Build history of the part. All positions in model axes, mm. Give positions to 0.01 mm unless a question says otherwise; leave off trailing zeros. Write each question's results on one line, items separated by ' | '. Start each with the question number.
1) Drill centre lines: line 1 along X through (y, z) = (1.3, 120); line 2 along Z through (x, y) = (104, 1.1). Where is each one in solid material? Low to high. Write a range as from..to.
2) Two-plate mould, pull along Y, no slides. Class faces 1 (the face through (-2, 2, -2)), 2 (the face through (-2, 0, -2)): +Y half, -Y half, draft (parallel to the pull), parting line (faces both ways), or undercut.
3) Drop a flat-ended pin along its axis: pin 1 Ø3 at (x, z) = (104, 120) entering from -Y. Give the stop position or say it passes through.
from build123d import *

# Parameters (mm, degrees)
SKETCH1_W                  = 220
SKETCH1_H                  = 280
BOSS_EXTRUDE1_DEPTH        = 2
F_3_5_3_5_DIAMETER_HOLE1_D = 3.5
FILLET1_R                  = 3


with BuildPart() as part:
    # Sketch1 → Boss-Extrude1 (new body)
    with BuildSketch(Plane(origin=(0, 0, 0), x_dir=(1, 0, 0), z_dir=(0, 1, 0))):
        Rectangle(SKETCH1_W, SKETCH1_H)
    extrude(amount=BOSS_EXTRUDE1_DEPTH)

    # Ø3.5 (3.5) Diameter Hole1 (through all)
    with Locations(Plane(origin=(0, 2, 0), x_dir=(1, 0, 0), z_dir=(0, 1, 0))):
        with Locations((-104, -120), (104, -120), (104, 120), (-104, 120), (104, 0), (-104, 0)):
            Hole(F_3_5_3_5_DIAMETER_HOLE1_D / 2)

    # Fillet1
    fillet1_edges = [part.edges().sort_by_distance(p)[0] for p in [
        (110, 1, 140),
        (-110, 1, 140),
        (-110, 1, -140),
        (110, 1, -140),
    ]]
    fillet(fillet1_edges, radius=FILLET1_R)


solid = part.part
Results:
1) line 1: -110..-105.75, -102.25..102.25, 105.75..110 | line 2: -140..-121.75, -118.25..-1.75, 1.75..118.25, 121.75..140
2) face 1: +Y half | face 2: -Y half
3) pin 1: through
